from build123d import *

# Parameters (mm, degrees)
SKETCH1_R           = 46
BOSS_EXTRUDE1_DEPTH = 38.5
SKETCH4_R           = 4
BOSS_EXTRUDE2_DEPTH = 12
SKETCH5_R           = 1.5
CUT_EXTRUDE1_DEPTH  = 6
CUT_EXTRUDE2_START  = -10
CUT_EXTRUDE2_DEPTH  = 10


with BuildPart() as part:
    # Sketch1 → Boss-Extrude1 (new body)
    with BuildSketch(Plane(origin=(0, 0, 0), x_dir=(1, 0, 0), z_dir=(0, 1, 0))):
        with Locations(Location((0, 0, 0), (0, 0, 270))):
            Circle(SKETCH1_R)
    extrude(amount=BOSS_EXTRUDE1_DEPTH)

    # Sketch2 → Cut-Revolve1 (revolve, cut)
    with BuildSketch(Plane.XY, mode=Mode.PRIVATE) as cut_revolve1_sk:
        with BuildLine():
            Line((-46, 38.5), (-46, 30.5))
            ThreePointArc((-46, 30.5), (-43.656854249, 36.156854249), (-38, 38.5))
            Line((-38, 38.5), (-46, 38.5))
        make_face()
    revolve(cut_revolve1_sk.sketch.rotate(Axis((0, 0, 0), (0, 1, 0)), 270), axis=Axis((0, 0, 0), (0, 1, 0)), mode=Mode.SUBTRACT)

    # Sketch3 → Cut-Revolve2 (revolve, cut)
    with BuildSketch(Plane.XY, mode=Mode.PRIVATE) as cut_revolve2_sk:
        Polygon((-46, 0), (-46, 4), (-31, 0), align=None)
    revolve(cut_revolve2_sk.sketch.rotate(Axis((0, 0, 0), (0, 1, 0)), 270), axis=Axis((0, 0, 0), (0, 1, 0)), mode=Mode.SUBTRACT)

    # Sketch4 → Boss-Extrude2 (add)
    with BuildSketch(Plane(origin=(0, 38.5, 0), x_dir=(1, 0, 0), z_dir=(0, 1, 0))):
        with Locations(Location((0, 0, 0), (0, 0, 270))):
            Circle(SKETCH4_R)
    extrude(amount=BOSS_EXTRUDE2_DEPTH)

    # Sketch5 → Cut-Extrude1 (cut)
    with BuildSketch(Plane(origin=(0, 38.5, 0), x_dir=(1, 0, 0), z_dir=(0, 1, 0))):
        with Locations(Location((-15.5, 0, 0), (0, 0, 270))):
            Circle(SKETCH5_R)
        with Locations(Location((0, 15.5, 0), (0, 0, 270))):
            Circle(SKETCH5_R)
        with Locations(Location((15.5, 0, 0), (0, 0, 270))):
            Circle(SKETCH5_R)
        with Locations(Location((0, -15.5, 0), (0, 0, 270))):
            Circle(SKETCH5_R)
    extrude(amount=-CUT_EXTRUDE1_DEPTH, mode=Mode.SUBTRACT)

    # Sketch6 → Cut-Extrude2 (cut)
    with BuildSketch(Plane(origin=(0, 50.5, 0), x_dir=(1, 0, 0), z_dir=(0, 1, 0)).offset(CUT_EXTRUDE2_START)):
        with BuildLine():
            Line((-3.249189343, 2.332974199), (2.894455289, 2.760820273))
            ThreePointArc((2.894455289, 2.760820273), (-0.277888697, 3.990335559), (-3.249189343, 2.332974199))
        make_face()
    extrude(amount=CUT_EXTRUDE2_DEPTH, mode=Mode.SUBTRACT)


solid = part.part
Verification items for the finished model (mm, model axes). A direction names the side the tool comes from. Give positions to 0.01 mm unless a question says otherwise; leave off trailing zeros. Write each loop counter-clockwise with the first axis right and the second up, starting at its lowest first coordinate (ties: lowest second). Pieces come first, ordered by that corner, then holes. Notation, with made-up numbers: M 35,78.5 L 45,78.5 A23 cw 45,108.5 Z; hole C 19,59 d5. An arc over 180 degrees is marked long. Write item = value, one per line.
(1) Sectioned sample at C-C (y = 16). Record the cut outline in (x, z), then the cut area to 3 significant figures.
Found:
outline = C 0,0 d92
area = 6,650 mm2
(2) Access from +Z, -Z, +X, -X, +Y, -Y to the whole of each face (thin tool, end or side, straight path). Record for faces 5 (the face through (38.787, 17.065, 24.729)), 6 (the face through (-15.05, 35.54, 1.43)).
Found:
face_5 = +Y, -Y
face_6 = +Y
(3) Sectioned sample at B-B (x = 0). Record the cut outline in (y, z).
Found:
outline = M 0,-31 L 4,-46 L 30.5,-46 A8 ccw 38.5,-38 L 38.5,-17 L 32.5,-17 L 32.5,-14 L 38.5,-14 L 38.5,-4 L 40.5,-4 L 40.5,-2.56 L 50.5,-2.56 L 50.5,4 L 38.5,4 L 38.5,14 L 32.5,14 L 32.5,17 L 38.5,17 L 38.5,38 A8 ccw 30.5,46 L 4,46 L 0,31 Z
(4) Draft check along X on faces 1 (the face through (-8, 38.5, -1)), 2 (the face through (-0.22, 45.43, -2.544)), 3 (the face through (0, 36, -17)), 4 (the face through (0, 32.5, 15)). Enter one of: released by +X, released by -X, zero draft, split by the parting line, or undercut.
Found:
face_1 = zero draft
face_2 = released by -X
face_3 = undercut
face_4 = undercut
(5) Material ranges on line 1 (X direction, y = 35.9, z = 0); line 2 (X direction, y = 36.9, z = 0); line 3 (Y direction, x = 17, z = 10.5), recorded low to high.
Found:
line_1 = -43.9 to -17, -14 to 14, 17 to 43.9
line_2 = -42.8 to -17, -14 to 14, 17 to 42.8
line_3 = 0 to 38.5
(6) Go/stop test with flat-tipped pins: pin 1 Ø3.5 at (x, z) = (-15, 0.5) entering from +Y; pin 2 Ø0.5 at (x, z) = (-1, -3.5) entering from +Y; pin 3 Ø10 at (y, z) = (32, -1.5) entering from -X. Record where each tip stops, or that it passes through.
Found:
pin_1 = 38.5
pin_2 = 40.5
pin_3 = -46
(7) Sectioned sample at A-A (z = 0). Record the cut outline in (x, y).
Found:
outline = M -46,4 L -31,0 L 31,0 L 46,4 L 46,30.5 A8 ccw 38,38.5 L 17,38.5 L 17,32.5 L 14,32.5 L 14,38.5 L 4,38.5 L 4,50.5 L -4,50.5 L -4,38.5 L -14,38.5 L -14,32.5 L -17,32.5 L -17,38.5 L -38,38.5 A8 ccw -46,30.5 Z
